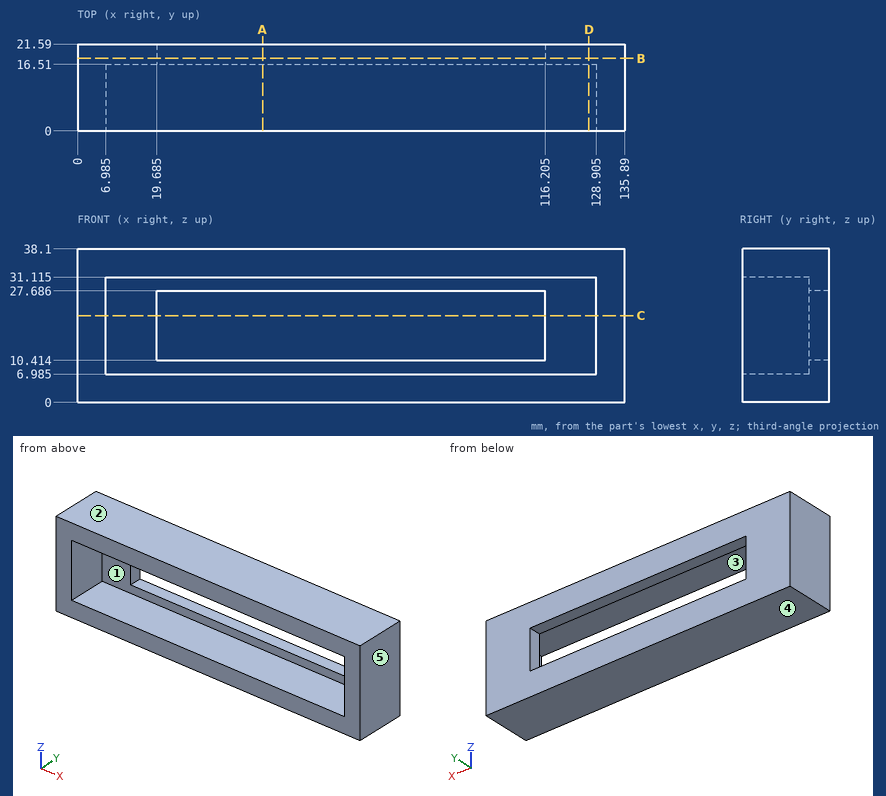
For this review, use the dimensioned drawing (mm, ordinates from the lowest corner) and the shaded views. A direction names the side the tool comes from. Give positions to 0.01 mm unless a question says otherwise; leave off trailing zeros. Order: outer loops, then holes, each group sorted by start corner. A loop starts at its lowest first (then second) coordinate and runs counter-clockwise, first axis right, second up.
1. For pin 1 Ø12 at (x, z) = (113.5, 20) entering from -Y, flat-tipped, find the tip position at first contact; note if it passes through.
Solution:
pin 1: stops at y = 16.51
2. Mouldability with a two-part tool opening along X and no side actions: class the marked faces 3, 4 and 5 as +X half, -X half, draft (parallel to the pull), parting line (faces both ways), or undercut.
Solution:
face 3: undercut
face 4: draft
face 5: +X half
3. Add section B-B, the plane y = 18. State the section outline as (x, z) points (3 decimals).
Solution:
outline: (0, 0) - (135.89, 0) - (135.89, 38.1) - (0, 38.1) - close; hole (19.685, 10.414) - (116.205, 10.414) - (116.205, 27.686) - (19.685, 27.686) - close
4. To check wall thickness, follow L1, parallel to Z at x = 64, y = 18.5; L2, parallel to Z at x = 47.5, y = 10.25 (3 decimals); L3, parallel to X at y = 11.5, z = 11.5 (3 decimals). State the ranges of each line that lie inside material, in increasing order.
Solution:
L1: z = 0 to 10.41, 27.69 to 38.1
L2: z = 0 to 6.985, 31.115 to 38.1
L3: x = 0 to 6.985, 128.905 to 135.89
5. Add section C-C, the plane z = 21.5. State the section outline as (x, y) points (3 decimals).
Solution:
outline: (0, 0) - (6.985, 0) - (6.985, 16.51) - (19.685, 16.51) - (19.685, 21.59) - (0, 21.59) - close; (116.205, 16.51) - (128.905, 16.51) - (128.905, 0) - (135.89, 0) - (135.89, 21.59) - (116.205, 21.59) - close
6. Add section D-D, the plane x = 127. State the section outline as (y, z) points (3 decimals).
Solution:
outline: (0, 0) - (21.59, 0) - (21.59, 38.1) - (0, 38.1) - (0, 31.115) - (16.51, 31.115) - (16.51, 6.985) - (0, 6.985) - close
7. Add section A-A, the plane x = 46. State the section outline as (y, z) points (3 decimals).
Solution:
outline: (0, 0) - (21.59, 0) - (21.59, 10.414) - (16.51, 10.414) - (16.51, 6.985) - (0, 6.985) - close; (0, 31.115) - (16.51, 31.115) - (16.51, 27.686) - (21.59, 27.686) - (21.59, 38.1) - (0, 38.1) - close
8. Tool access review of the marked faces 1 and 2: name each direction out of +Z, -Z, +X, -X, +Y, -Y from which nothing blocks a thin tool from reaching the whole face with its end or side.
Solution:
face 1: -Y
face 2: +Z, +X, -X, +Y, -Y
